from build123d import *

# Parameters (mm, degrees)
SKETCH_1_R      = 27
SKETCH_1_R_2    = 24
EXTRUDE_1_DEPTH = 28
EXTRUDE_2_DEPTH = 15
SKETCH_3_R      = 8
EXTRUDE_3_DEPTH = 6
SKETCH_4_R      = 17.5
EXTRUDE_4_DEPTH = 6


with BuildPart() as part:
    # 草图1 → 凸台-拉伸1 (new body)
    with BuildSketch(Plane.XY):
        Circle(SKETCH_1_R)
        Circle(SKETCH_1_R_2, mode=Mode.SUBTRACT)
    extrude(amount=EXTRUDE_1_DEPTH)

    # 草图2 → 凸台-拉伸2 (add)
    with BuildSketch(Plane.XY):
        with BuildLine():
            Line((-2, 25.5), (-3.56, 9.26))
            ThreePointArc((-3.56, 9.26), (-5.831268155, 8.026052062), (-7.706682841, 6.247258566))
            Line((-7.706682841, 6.247258566), (-23.633907177, 9.782046389))
            Line((-23.633907177, 9.782046389), (-24.869975154, 5.977820324))
            Line((-24.869975154, 5.977820324), (-9.906883841, -0.52426383))
            ThreePointArc((-9.906883841, -0.52426383), (-9.435190072, -3.065679092), (-8.322991936, -5.39898187))
            Line((-8.322991936, -5.39898187), (-16.606557922, -19.454362852))
            Line((-16.606557922, -19.454362852), (-13.370489945, -21.805503861))
            Line((-13.370489945, -21.805503861), (-2.562790936, -9.584012866))
            ThreePointArc((-2.562790936, -9.584012866), (0, -9.92074594), (2.562790936, -9.584012866))
            Line((2.562790936, -9.584012866), (13.370489945, -21.805503861))
            Line((13.370489945, -21.805503861), (16.606557922, -19.454362852))
            Line((16.606557922, -19.454362852), (8.322991936, -5.39898187))
            ThreePointArc((8.322991936, -5.39898187), (9.435190072, -3.065679092), (9.906883841, -0.52426383))
            Line((9.906883841, -0.52426383), (24.869975154, 5.977820324))
            Line((24.869975154, 5.977820324), (23.633907177, 9.782046389))
            Line((23.633907177, 9.782046389), (7.706682841, 6.247258566))
            ThreePointArc((7.706682841, 6.247258566), (5.831268155, 8.026052062), (3.56, 9.26))
            Line((3.56, 9.26), (2, 25.5))
            Line((2, 25.5), (-2, 25.5))
        make_face()
    extrude(amount=EXTRUDE_2_DEPTH)

    # 草图3 → 凸台-拉伸3 (add)
    with BuildSketch(Plane.XY.offset(15)):
        Circle(SKETCH_3_R)
        Polygon((3.560842768, -5.943096733), (6.927294132, 0.11223193), (3.366451364, 6.055328663), (-3.560842768, 5.943096733), (-6.927294132, -0.11223193), (-3.366451364, -6.055328663), align=None, mode=Mode.SUBTRACT)
    extrude(amount=EXTRUDE_3_DEPTH)

    # 草图4 → 凸台-拉伸4 (add)
    with BuildSketch(Plane(origin=(0, 0, 0), x_dir=(-1, 0, 0), z_dir=(0, 0, -1))):
        Circle(SKETCH_4_R)
    extrude(amount=-EXTRUDE_4_DEPTH)


solid = part.part
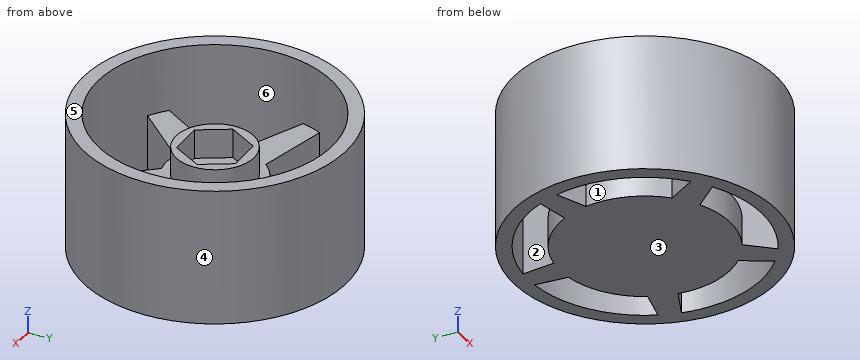
Verification items for the finished model (mm, model axes). Face numbers are marked on the shaded views. A direction names the side the tool comes from. Coordinates: 2 decimals unless noted, no trailing zeros. Loops run counter-clockwise (first coordinate to the right, second up) from the corner with the lowest first, then second, coordinate; pieces in that order, holes last. Notation, with made-up numbers: M -20.75,42.25 L -13.75,42.25 A33 cw -13.75,76.25 Z; hole C -34,-9 d9. An arc over 180 degrees is marked long. One line per item, written item: value.
1. Set-up check for the marked faces 1, 2 and 3: record each of +Z, -Z, +X, -X, +Y, -Y from which the full face is reachable in a straight line by a thin tool's end or side.
Answers follow:
face 1: +Z, -Z
face 2: +Z
face 3: -Z, +X, -X, +Y, -Y
2. Section check B-B on z = 13.75. Record the cut outline in (x, y), plus the area to 3 significant figures.
Answers follow:
outline: C 0,0 d54; hole M -23.4,5.34 A24 ccw -15.79,-18.07 L -8.32,-5.4 A9.92 cw -9.91,-0.52 Z; hole M -22.07,9.43 L -7.71,6.25 A9.92 cw -3.56,9.26 L -2.15,23.9 A24 ccw Z; hole M -12.31,-20.6 A24 ccw 12.31,-20.6 L 2.56,-9.58 A9.92 cw -2.56,-9.58 Z; hole M 2.15,23.9 L 3.56,9.26 A9.92 cw 7.71,6.25 L 22.07,9.43 A24 ccw Z; hole M 8.32,-5.4 L 15.79,-18.07 A24 ccw 23.4,5.34 L 9.91,-0.52 A9.92 cw Z
area: 1,190 mm^2
3. Gauge pin test, flat ends, axial feed: P1, Ø9, axis at x = 6.5, y = 14, coming from the +Z side; P2, Ø4, axis at x = 11, z = 19.5, coming from the -Y side; P3, Ø10, axis at y = -12, z = 10.5, coming from the +X side; P4, Ø3, axis at x = 12, y = 16.5, coming from the -Z side. Record the tip position at first contact, or that the pin passes through.
Answers follow:
P1: z = 15
P2: y = -25.46
P3: x = 26.08
P4: through
4. Material ranges on line 1 along Y through (x, z) = (-0.5, 26.75); line 2 along Y through (x, z) = (0, 9.75); line 3 along X through (y, z) = (-8.5, 2.75), recorded low to high. Write a range as from..to.
Answers follow:
line 1: -27..-23.99, 23.99..27
line 2: -27..-24, -9.92..27
line 3: -25.63..-22.44, -15.3..15.3, 22.44..25.63
5. Section check A-A on z = 17.25. Record the cut outline in (x, y).
Answers follow:
outline: C 0,0 d54; C 0,0 d16; hole C 0,0 d48; hole M -6.93,-0.11 L -3.37,-6.06 L 3.56,-5.94 L 6.93,0.11 L 3.37,6.06 L -3.56,5.94 Z
6. Mould release check, pull along Y, two halves, no side actions. Record for the marked faces 4, 5 and 6: pulls with the +Y half, pulls with the -Y half, needs draft (parallel to the pull), parting line crosses it, or undercut.
Answers follow:
face 4: parting line crosses it
face 5: needs draft
face 6: undercut
7. Section check D-D on x = -20. Record the cut outline in (y, z).
Answers follow:
outline: M -18.14,0 L -13.27,0 L -13.27,28 L -18.14,28 Z; M 3.86,0 L 8.98,0 L 8.98,15 L 3.86,15 Z; M 13.27,0 L 18.14,0 L 18.14,28 L 13.27,28 Z
8. Section check C-C on x = 0. Record the cut outline in (y, z).
Answers follow:
outline: M -27,0 L -24,0 L -24,28 L -27,28 Z; M -17.5,0 L 27,0 L 27,28 L 24,28 L 24,15 L 8,15 L 8,21 L 6,21 L 6,15 L -6,15 L -6,21 L -8,21 L -8,15 L -9.92,15 L -9.92,6 L -17.5,6 Z
